Solid Edge part; units mm, degrees
sketch "Sketch1" plane through (0, 0, 0) normal (0, -1, 0) x (1, 0, 0)
  line L0 (-2.05, 37.3) -> (-2.05, -37.3)
  arc A0 (-2.05, -37.3) -> (-9.05, -44.3) centre (-9.05, -37.3) cw
  line L1 (-27.5, -44.3) -> (-9.05, -44.3)
  line L2 (-27.5, -50) -> (-27.5, -44.3)
  line L3 (27.5, -50) -> (-27.5, -50)
  line L4 (27.5, -50) -> (27.5, -44.3)
  line L5 (27.5, -44.3) -> (9.05, -44.3)
  arc A1 (2.05, -37.3) -> (9.05, -44.3) centre (9.05, -37.3) ccw
  line L6 (2.05, -37.3) -> (2.05, 37.3)
  arc A2 (9.05, 44.3) -> (2.05, 37.3) centre (9.05, 37.3) ccw
  line L7 (27.5, 44.3) -> (9.05, 44.3)
  line L8 (27.5, 50) -> (27.5, 44.3)
  line L9 (-27.5, 50) -> (27.5, 50)
  line L10 (-27.5, 44.3) -> (-27.5, 50)
  line L11 (-27.5, 44.3) -> (-9.05, 44.3)
  arc A3 (-9.05, 44.3) -> (-2.05, 37.3) centre (-9.05, 37.3) cw
  dimension "D1" = 27.5
  dimension "D2" = 27.5
extrude "Protrusion1" add sketch "Sketch1" against normal blind 41.275
Verification items for the finished model (mm, model axes). A direction names the side the tool comes from. Coordinates: 2 decimals unless noted, no trailing zeros. Order: outer loops, then holes, each group sorted by start corner. A loop starts at its lowest first (then second) coordinate and runs counter-clockwise, first axis right, second up. Notation, with made-up numbers: (8, 13.25) -> (52, 13.25) arc R15 cw to (52, 33.25) -> close; hole circle Ø2 at (8, -35.5). An arc over 180 degrees is marked (long way). Use CSV: the item, a comma, the result in double quotes. Start each with the question number.
Q1. Section check B-B, the plane y = 9.5. Record the cut outline in (x, z).
Q2. Thickness scan on line 1 along Z through (x, y) = (25, 36); line 2 along X through (y, z) = (35, -16); line 3 along Z through (x, y) = (-7, 11). Record the ranges inside material, lowest first.
Q3. Section check D-D, the plane z = -15.5. Record the cut outline in (x, y) (3 decimals), and give its area (3 significant figures).
Q4. Section check A-A, the plane x = 23.5. Record the cut outline in (y, z) (3 decimals), and give its area (3 significant figures).
Q5. Section check C-C, the plane x = -5.5. Record the cut outline in (y, z) (3 decimals).
Q6. Tool access check on faces 4 (the cylindrical face through (4.05, 20.35, -42.2)), 5 (the flat face through (-18, 20, -44.3)), 6 (the flat face through (-27.5, 20, -47)). Record the directions out of +Z, -Z, +X, -X, +Y, -Y that give a thin tool (end or side, any length) a straight path to the whole face; none if there is none.
Q7. Depth check by flat-ended pin: P1, Ø4, axis at y = 23.5, z = -30.5, coming from the +X side; P2, Ø3, axis at y = 33, z = 3, coming from the -X side; P3, Ø6, axis at x = -12.5, z = -39, coming from the -Y side. Enter the tip coordinate at first touch or a pass-through.
Q8. Draft check along Z on faces 1 (the cylindrical face through (4.15, 20.35, 42.3)), 2 (the flat face through (0, 20, 50)), 3 (the flat face through (0, 0, 8)). Enter one of: +Z half, -Z half, draft (parallel to the pull), parting line (faces both ways), or undercut.
Returned:
1,outline,"(-27.5, -50) -> (27.5, -50) -> (27.5, -44.3) -> (9.05, -44.3) arc R7 cw to (2.05, -37.3) -> (2.05, 37.3) arc R7 cw to (9.05, 44.3) -> (27.5, 44.3) -> (27.5, 50) -> (-27.5, 50) -> (-27.5, 44.3) -> (-9.05, 44.3) arc R7 cw to (-2.05, 37.3) -> (-2.05, -37.3) arc R7 cw to (-9.05, -44.3) -> (-27.5, -44.3) -> close"
2,line 1,"z = -50 to -44.3, 44.3 to 50"
2,line 2,"x = -2.05 to 2.05"
2,line 3,"z = -50 to -43.99, 43.99 to 50"
3,outline,"(-2.05, 0) -> (2.05, 0) -> (2.05, 41.275) -> (-2.05, 41.275) -> close"
3,area,"169 mm^2"
4,outline,"(0, -50) -> (41.275, -50) -> (41.275, -44.3) -> (0, -44.3) -> close; (0, 44.3) -> (41.275, 44.3) -> (41.275, 50) -> (0, 50) -> close"
4,area,"471 mm^2"
5,outline,"(0, -50) -> (41.275, -50) -> (41.275, -43.333) -> (0, -43.333) -> close; (0, 43.333) -> (41.275, 43.333) -> (41.275, 50) -> (0, 50) -> close"
6,face 4,"+X, +Y, -Y"
6,face 5,"-X, +Y, -Y"
6,face 6,"+Z, -Z, -X, +Y, -Y"
7,P1,"stops at x = 2.05"
7,P2,"stops at x = -2.05"
7,P3,"passes through"
8,face 1,"undercut"
8,face 2,"+Z half"
8,face 3,"draft"
